Here's how the part is built. I have some questions about the finished solid (model axes, mm). A direction names the side the tool comes from. Coordinates: 2 decimals unless noted, no trailing zeros. Write each loop counter-clockwise with the first axis right and the second up, starting at its lowest first coordinate (ties: lowest second). Pieces come first, ordered by that corner, then holes.
```python
from build123d import *

# Parameters (mm, degrees)
SKETCH2_W           = 80
SKETCH2_H           = 50
SKETCH2_R           = 2
BOSS_EXTRUDE1_DEPTH = 1.5
BOSS_EXTRUDE2_DEPTH = 17.5
SKETCH2_5_W         = 12
SKETCH2_5_H         = 4
BOSS_EXTRUDE3_DEPTH = 4


with BuildPart() as part:
    # Sketch2 → Boss-Extrude1 (new body)
    with BuildSketch(Plane(origin=(0, 0, 0), x_dir=(1, 0, 0), z_dir=(0, 1, 0))):
        with Locations((40, -25)):
            Rectangle(SKETCH2_W, SKETCH2_H)
        with Locations((53.5, -46)):
            Circle(SKETCH2_R, mode=Mode.SUBTRACT)
    extrude(amount=BOSS_EXTRUDE1_DEPTH)

    # Sketch2<3> → Boss-Extrude2 (add)
    with BuildSketch(Plane(origin=(0, 0, 0), x_dir=(1, 0, 0), z_dir=(0, 1, 0))):
        Polygon((47.407334239, -36.646178921), (61.72925499, -49), (77.292723547, -49), (77.292723547, -38.583095808), (59.246513421, -26), (59.246513421, -1), (15.322098265, -1), (15.322098265, -49), (36.751159142, -49), align=None)
    extrude(amount=BOSS_EXTRUDE2_DEPTH)

    # Sketch2<5> → Boss-Extrude3 (add)
    with BuildSketch(Plane(origin=(0, 0, 0), x_dir=(1, 0, 0), z_dir=(0, 1, 0))):
        with Locations((66.923917494, -4.397775479)):
            Rectangle(SKETCH2_5_W, SKETCH2_5_H)
    extrude(amount=BOSS_EXTRUDE3_DEPTH)


solid = part.part
```
1) Imagine slicing it at B-B on z = 46. Please give me the cut outline in (x, y), then the cut area to 3 significant figures.
Values follow:
outline: (0, 0) - (51.5, 0) - (51.5, 1.5) - (39.34, 1.5) - (39.34, 17.5) - (15.32, 17.5) - (15.32, 1.5) - (0, 1.5) - close; (55.5, 0) - (80, 0) - (80, 1.5) - (77.29, 1.5) - (77.29, 17.5) - (58.25, 17.5) - (58.25, 1.5) - (55.5, 1.5) - close
area: 803 mm2
2) Imagine slicing it at C-C on y = 10.75. Please give me the cut outline in (x, z).
Values follow:
outline: (15.32, 1) - (59.25, 1) - (59.25, 26) - (77.29, 38.58) - (77.29, 49) - (61.73, 49) - (47.41, 36.65) - (36.75, 49) - (15.32, 49) - close
3) I need wall thicknesses on probe 1 along X at (y, z) = (0.6, 46); probe 2 along Z at (x, y) = (53.5, 0.6); probe 3 along Z at (x, y) = (21, 16.25). Which ranges of each line are inside material? Lowest first, please.
Values follow:
probe 1: x = 0 to 51.5, 55.5 to 80
probe 2: z = 0 to 44, 48 to 50
probe 3: z = 1 to 49
4) Will these pins go through, and if not, where does the flat tip stop? pin 1 (10 mm diameter, centred on x = 68.5, y = 12, fed in from +Z); pin 2 (8 mm diameter, centred on y = 12.5, z = 30, fed in from -X); pin 3 (8 mm diameter, centred on x = 45.5, y = 9, fed in from +Z); pin 4 (3 mm diameter, centred on x = 53.5, z = 46, fed in from +Y).
Values follow:
pin 1: stops at z = 49
pin 2: stops at x = 15.32
pin 3: stops at z = 43.49
pin 4: passes through
5) Imagine slicing it at A-A on x = 52.5. Please give me the cut outline in (y, z), then the cut area to 3 significant figures.
Values follow:
outline: (0, 0) - (1.5, 0) - (1.5, 1) - (17.5, 1) - (17.5, 41.04) - (1.5, 41.04) - (1.5, 44.27) - (0, 44.27) - close; (0, 47.73) - (1.5, 47.73) - (1.5, 50) - (0, 50) - close
area: 710 mm2
6) On a 3-axis mill with a long thin cutter (end or side, diameter ignored), from which of +Z, -Z, +X, -X, +Y, -Y can I reach the whole of each face in a straight line? I mean faces 4 (the face through (15.322, 9, 25)), 5 (the face through (69, 9, 49)), 6 (the face through (42.005, 9.388, 42.91)), 7 (the face through (77.293, 9, 44)), 8 (the face through (67, 3, 2.398)). Say none if no direction works.
Values follow:
face 4: +Z, -Z, -X, +Y
face 5: +Z, +X, -X, +Y
face 6: +Z, +Y
face 7: +Z, -Z, +X, +Y
face 8: -Z, +X, +Y
7) We'd pull the mould along Z, two halves only. Please class faces 1 (the face through (39, 1, 0)), 2 (the face through (53.066, 0.74, 47.952)), 3 (the face through (39, 17.5, 25)): pulls with the +Z half, pulls with the -Z half, needs draft (parallel to the pull), parting line crosses it, or undercut.
Values follow:
face 1: pulls with the -Z half
face 2: undercut
face 3: needs draft
8) Imagine slicing it at D-D on z = 19. Please give me the cut outline in (x, y), then the cut area to 3 significant figures.
Values follow:
outline: (0, 0) - (80, 0) - (80, 1.5) - (59.25, 1.5) - (59.25, 17.5) - (15.32, 17.5) - (15.32, 1.5) - (0, 1.5) - close
area: 823 mm2
